The listing builds one solid part. Answer for the finished solid, in the listing's coordinates (mm). A direction names the side the tool comes from. Coordinates: 2 decimals unless noted, no trailing zeros. Write each loop counter-clockwise with the first axis right and the second up, starting at its lowest first coordinate (ties: lowest second). Pieces come first, ordered by that corner, then holes.
(1) The part is cut by section A-A on z = 11. Determine the outline of the cut face in (x, y), plus the area to 3 significant figures.
(2) Given P1, Ø5, axis at x = 0, z = 22.5, coming from the -Y side; P2, Ø3, axis at y = 1, z = 14, coming from the +X side; P3, Ø6, axis at x = 0.5, z = 16.5, coming from the -Y side, each flat-ended and moving along its own axis, determine where each tip first touches the part or whether it passes through.
(3) The part is cut by section C-C on y = -5. Determine the outline of the cut face in (x, z).
(4) The part is cut by section B-B on x = 0. Give the number of separate pieces and of enclosed holes in the cut face, plus the area to 3 significant figures.
(5) For a pull along Z with two mould halves and no side action, classify faces 6 (the flat face through (6.844, -3.774, 23.011)), 7 (the flat face through (3, -1.5, 3)), 8 (the flat face through (-6.4, 3.5, 9.6)), 9 (the flat face through (0, -1, 26)) as +Z half, -Z half, draft (parallel to the pull), parting line (faces both ways), or undercut.
(6) Straight lines are drawn through the part: line 1 (X direction, y = 2.75, z = 11); line 2 (X direction, y = 1.35, z = 19); line 3 (Z direction, x = 2.25, y = -0.5). For each, find the intervals that lie inside material, in ascending order.
(7) Which of the six approach directions +Z, -Z, +X, -X, +Y, -Y give full straight-line access (tool end or side, diameter ignored) to faces 1 (the flat face through (-3, 2, 24)), 2 (the flat face through (7.4, 1.5, 16.5)), 3 (the flat face through (7, -4, 23.8)), 4 (the conical face through (-7.37, 3.51, 18.09)), 5 (the flat face through (-3.76, -3.77, 24.92))?
from build123d import *
from build123d.topology import SkipClean

# Parameters (mm, degrees)
EXTRUDE_1_DEPTH        = 4
EXTRUDE_3_DEPTH        = 6
CHAMFER_1_SIZE         = 3
SKETCH_5_R             = 0.85
CUT_EXTRUDE_1_DEPTH    = 4
PATTERN_LINEAR_1_COUNT = 2
PATTERN_LINEAR_1_PITCH = 8
CUT_EXTRUDE_2_DEPTH    = 2.5
CUT_EXTRUDE_3_REACH    = 30.061
SKETCH_7_R             = 1.35
SKETCH_8_R             = 6
EXTRUDE_4_DEPTH        = 1.5
FILLET_1_R             = 0.5
SKETCH_9_R             = 5
CUT_EXTRUDE_4_DEPTH    = 3.6
SKETCH_10_R            = 3.55
CUT_EXTRUDE_5_DEPTH    = 3.6
CUT_EXTRUDE_6_DEPTH    = 0.8
CUT_EXTRUDE_7_DEPTH    = 29.786455148
FILLET_2_R             = 2
CHAMFER_2_SIZE         = 1


with BuildPart() as part:
    # ｽｹｯﾁ1 → ﾎﾞｽ - 押し出し1 (new body)
    with BuildSketch(Plane(origin=(0, 0, 0), x_dir=(1, 0, 0), z_dir=(0, 1, 0))):
        with BuildLine():
            Line((-7.9, 0), (-7.9, -26))
            Line((-7.9, -26), (7.9, -26))
            Line((7.9, -26), (7.9, 0))
            ThreePointArc((7.9, 0), (0, 7.9), (-7.9, 0))
        make_face()
    extrude(amount=EXTRUDE_1_DEPTH)

    # ｽｹｯﾁ4 → ﾎﾞｽ - 押し出し3 (add)
    with BuildSketch(Plane.XY.offset(26)):
        Polygon((-7, -5.5), (-4.5, -5.5), (-3, -2), (3, -2), (4.5, -5.5), (7, -5.5), (7.9, -2), (7.9, 0), (-7.9, 0), (-7.9, -2), align=None)
    extrude(amount=-EXTRUDE_3_DEPTH)

    # 面取り1
    chamfer_1_edges = [part.edges().sort_by_distance(p)[0] for p in [
        (0, 4, 26),
    ]]
    chamfer(chamfer_1_edges, length=CHAMFER_1_SIZE)

    # ｽｹｯﾁ5 → ｶｯﾄ - 押し出し1 (cut)
    with BuildSketch(Plane(origin=(0, 4, 0), x_dir=(1, 0, 0), z_dir=(0, 1, 0))):
        with Locations(Location((-4, -19, 0), (0, 0, 270))):
            Circle(SKETCH_5_R)
        with Locations(Location((4, -19, 0), (0, 0, 270))):
            Circle(SKETCH_5_R)
    cut_extrude_1 = extrude(amount=-CUT_EXTRUDE_1_DEPTH, mode=Mode.SUBTRACT)

    # 直線ﾊﾟﾀｰﾝ1: ｶｯﾄ - 押し出し1 ×2
    with Locations(*[(0, 0, -i * PATTERN_LINEAR_1_PITCH) for i in range(1, PATTERN_LINEAR_1_COUNT)]):
        add(cut_extrude_1, mode=Mode.SUBTRACT)

    # ｽｹｯﾁ6 → ｶｯﾄ - 押し出し2 (cut)
    with BuildSketch(Plane(origin=(0, 4, 0), x_dir=(1, 0, 0), z_dir=(0, 1, 0))):
        with BuildLine():
            Line((-3, -23), (-3, -27))
            Line((-3, -27), (3, -27))
            Line((3, -27), (3, -23))
            ThreePointArc((3, -23), (0, -20), (-3, -23))
        make_face()
    extrude(amount=-CUT_EXTRUDE_2_DEPTH, mode=Mode.SUBTRACT)

    # ｽｹｯﾁ7 → ｶｯﾄ - 押し出し3 (cut, up to next)
    with BuildSketch(Plane(origin=(0, 1.5, 0), x_dir=(1, 0, 0), z_dir=(0, 1, 0)), mode=Mode.PRIVATE) as cut_extrude_3_sk1:
        with Locations(Location((0, -23, 0), (0, 0, 270))):
            Circle(SKETCH_7_R)
    cut_extrude_3_tool1 = extrude(cut_extrude_3_sk1.sketch, amount=-CUT_EXTRUDE_3_REACH, mode=Mode.PRIVATE) & part.part
    add(cut_extrude_3_tool1.solids().sort_by_distance((0, 1.5, 23))[0], mode=Mode.SUBTRACT)

    # ｽｹｯﾁ8 → ﾎﾞｽ - 押し出し4 (add)
    with BuildSketch(Plane.XZ):
        with Locations(Location((0, 0, 0), (0, 0, 90))):
            Circle(SKETCH_8_R)
    extrude(amount=EXTRUDE_4_DEPTH)

    # ﾌｨﾚｯﾄ1
    fillet_1_edges = [part.edges().sort_by_distance(p)[0] for p in [
        (0, 0, -6),
    ]]
    fillet(fillet_1_edges, radius=FILLET_1_R)

    # ｽｹｯﾁ9 → ｶｯﾄ - 押し出し4 (cut)
    with BuildSketch(Plane(origin=(0, 4, 0), x_dir=(1, 0, 0), z_dir=(0, 1, 0))):
        with Locations(Location((0, 0, 0), (0, 0, 270))):
            Circle(SKETCH_9_R)
    extrude(amount=-CUT_EXTRUDE_4_DEPTH, mode=Mode.SUBTRACT)

    # ｽｹｯﾁ10 → ｶｯﾄ - 押し出し5 (cut)
    with BuildSketch(Plane(origin=(0, 0.4, 0), x_dir=(1, 0, 0), z_dir=(0, 1, 0))):
        with Locations(Location((0, 0, 0), (0, 0, 270))):
            Circle(SKETCH_10_R)
    extrude(amount=-CUT_EXTRUDE_5_DEPTH, mode=Mode.SUBTRACT)

    # ｽｹｯﾁ11 → ｶｯﾄ - 押し出し6 (cut, symmetric)
    with BuildSketch(Plane.XY.offset(23)):
        Polygon((3, -2), (4.5, -5.5), (5.1, -5.5), (3.6, -2), align=None)
        Polygon((7.9, -2), (7, -5.5), (6.4, -5.5), (7.3, -2), align=None)
    cut_extrude_6 = extrude(amount=CUT_EXTRUDE_6_DEPTH, both=True, mode=Mode.SUBTRACT)

    # ﾐﾗｰ1: ｶｯﾄ - 押し出し6 across plane
    add(cut_extrude_6.mirror(Plane(origin=(0, 0, 0), x_dir=(0, 0, 1), z_dir=(1, 0, 0))), mode=Mode.SUBTRACT)

    # ｽｹｯﾁ12 → ｶｯﾄ - 押し出し7 (cut, through all)
    with SkipClean():  # the faces are left unmerged after this step: merging them gives an invalid solid
        with BuildSketch(Plane(origin=(0, 4, 0), x_dir=(1, 0, 0), z_dir=(0, 1, 0))):
            with BuildLine():
                Line((-7.9, -18), (-6.9, -15))
                Line((-6.9, -15), (-6.9, -3.847076812))
                ThreePointArc((-6.9, -3.847076812), (-7.645913941, -1.987460691), (-7.9, 0))
                Line((-7.9, 0), (-7.9, -18))
            make_face()
        cut_extrude_7 = extrude(amount=-CUT_EXTRUDE_7_DEPTH, mode=Mode.SUBTRACT)

    # ﾐﾗｰ2: ｶｯﾄ - 押し出し7 across plane
    with SkipClean():  # the faces are left unmerged after this step: merging them gives an invalid solid
        add(cut_extrude_7.mirror(Plane(origin=(0, 0, 0), x_dir=(0, 0, 1), z_dir=(1, 0, 0))), mode=Mode.SUBTRACT)

    # ﾌｨﾚｯﾄ2
    fillet_2_edges = [part.edges().sort_by_distance(p)[0] for p in [
        (-7.9, 2, 18),
        (-6.9, 2, 3.847076812),
        (-6.9, 2, 15),
        (7.9, 2, 18),
        (6.9, 2, 15),
        (6.9, 2, 3.847076812),
    ]]
    fillet(fillet_2_edges, radius=FILLET_2_R)

    # 面取り2
    # the kernel refuses this chamfer: 1 mm, written as the material it adds along each edge
    with BuildSketch(Plane(origin=(7.9, 0, 20), x_dir=(0, 0.02749587661058639, -0.9996219169112968), z_dir=(-1, 0, 0))) as chamfer_2_piece_1_section:
        Polygon((CHAMFER_2_SIZE * 0.999621916911, CHAMFER_2_SIZE * 0.0274958766106), (-CHAMFER_2_SIZE * 0.0274958766106, CHAMFER_2_SIZE * 0.999621916911), (0, 0), align=None)
    chamfer_2_piece_1 = extrude(amount=15.8, mode=Mode.PRIVATE)
    chamfer_2_piece_1 = chamfer_2_piece_1 - Plane(origin=(-4, -0.34097177, 19), x_dir=(0, 0, 1), z_dir=(0, 1, 0)) * Cylinder(0.85, 36, mode=Mode.PRIVATE)
    chamfer_2_piece_1 = chamfer_2_piece_1 - Plane(origin=(4, -0.34097177, 19), x_dir=(0, 0, 1), z_dir=(0, 1, 0)) * Cylinder(0.85, 36, mode=Mode.PRIVATE)
    add(chamfer_2_piece_1)
    # the kernel refuses this chamfer: 1 mm, written as the material it takes off along each edge
    with BuildSketch(Plane(origin=(-7.9, 4, 18.32455532), x_dir=(-0.027495876610586487, -0.9996219169112968, 0), z_dir=(0, 0, 1)), Plane(origin=(7.9, 4, 25.571682988), x_dir=(0.027495876610586487, -0.9996219169112968, 0), z_dir=(0, 0, -1))) as chamfer_2_2_piece_1:
        Polygon((CHAMFER_2_SIZE * 0.999621916911, CHAMFER_2_SIZE * 0.0274958766106), (-CHAMFER_2_SIZE * 0.0274958766106, CHAMFER_2_SIZE * 0.999621916911), (0, 0), align=None)
    extrude(amount=7.247127668, mode=Mode.SUBTRACT)
    with BuildSketch(Plane(origin=(0, 4, 0), x_dir=(1, 0, 0), z_dir=(0, 0, 1))) as chamfer_2_2_piece_2:
        Polygon((7.9, -CHAMFER_2_SIZE), (7.9 - CHAMFER_2_SIZE, 0), (7.9, 0), align=None)
    revolve(axis=Axis((0, 4, 0), (0, 1, 0)), revolution_arc=180, mode=Mode.SUBTRACT)
    with BuildSketch(Plane(origin=(-5.9, 4, 18.32455532), x_dir=(-1, 0, 0), z_dir=(0, 0, 1))) as chamfer_2_2_piece_3:
        Polygon((2, CHAMFER_2_SIZE), (2 - CHAMFER_2_SIZE, 0), (2, 0), align=None)
    revolve(axis=Axis((-5.9, 4, 18.32455532), (0, -1, 0)), revolution_arc=18.434948823, mode=Mode.SUBTRACT)
    with BuildSketch(Plane(origin=(-7.797366596, 4, 17.692099788), x_dir=(-0.026084878905720917, -0.9996219169112968, -0.008694959635240323), z_dir=(0.31622776601683844, 0, -0.9486832980505137))) as chamfer_2_2_piece_4:
        Polygon((CHAMFER_2_SIZE * 0.999621916911, -CHAMFER_2_SIZE * 0.0274958766106), (-CHAMFER_2_SIZE * 0.0274958766106, -CHAMFER_2_SIZE * 0.999621916911), (0, 0), align=None)
    extrude(amount=2.513167019, mode=Mode.SUBTRACT)
    with BuildSketch(Plane(origin=(-8.9, 4, 14.67544468), x_dir=(0.9486832980505138, 0, 0.31622776601683794), z_dir=(-0.31622776601683794, 0, 0.9486832980505138))) as chamfer_2_2_piece_5:
        Polygon((2, -CHAMFER_2_SIZE), (2 + CHAMFER_2_SIZE, 0), (2, 0), align=None)
    revolve(axis=Axis((-8.9, 4, 14.67544468), (0, 1, 0)), revolution_arc=18.434948823, mode=Mode.SUBTRACT)
    with BuildSketch(Plane(origin=(-6.9, 4, 14.67544468), x_dir=(-0.027495876610586487, -0.9996219169112968, 0), z_dir=(0, 0, -1))) as chamfer_2_2_piece_6:
        Polygon((CHAMFER_2_SIZE * 0.999621916911, -CHAMFER_2_SIZE * 0.0274958766106), (-CHAMFER_2_SIZE * 0.0274958766106, -CHAMFER_2_SIZE * 0.999621916911), (0, 0), align=None)
    extrude(amount=10.339548002, mode=Mode.SUBTRACT)
    with BuildSketch(Plane(origin=(-8.9, 4, 4.335896678), x_dir=(1, 0, 0), z_dir=(0, 0, 1))) as chamfer_2_2_piece_7:
        Polygon((2, -CHAMFER_2_SIZE), (2 + CHAMFER_2_SIZE, 0), (2, 0), align=None)
    revolve(axis=Axis((-8.9, 4, 4.335896678), (0, 1, 0)), revolution_arc=25.974390018, mode=Mode.SUBTRACT)
    with BuildSketch(Plane(origin=(8.9, 4, 4.335896678), x_dir=(-0.8989898989898989, 0, -0.43796936138745074), z_dir=(0.43796936138745074, 0, -0.8989898989898989))) as chamfer_2_2_piece_8:
        Polygon((2, -CHAMFER_2_SIZE), (2 + CHAMFER_2_SIZE, 0), (2, 0), align=None)
    revolve(axis=Axis((8.9, 4, 4.335896678), (0, 1, 0)), revolution_arc=25.974390018, mode=Mode.SUBTRACT)
    with BuildSketch(Plane(origin=(6.9, 4, 14.67544468), x_dir=(0.027495876610586487, -0.9996219169112968, 0), z_dir=(0, 0, -1))) as chamfer_2_2_piece_9:
        Polygon((CHAMFER_2_SIZE * 0.999621916911, CHAMFER_2_SIZE * 0.0274958766106), (-CHAMFER_2_SIZE * 0.0274958766106, CHAMFER_2_SIZE * 0.999621916911), (0, 0), align=None)
    extrude(amount=10.339548002, mode=Mode.SUBTRACT)
    with BuildSketch(Plane(origin=(8.9, 4, 14.67544468), x_dir=(-1, 0, 0), z_dir=(0, 0, -1))) as chamfer_2_2_piece_10:
        Polygon((2, -CHAMFER_2_SIZE), (2 + CHAMFER_2_SIZE, 0), (2, 0), align=None)
    revolve(axis=Axis((8.9, 4, 14.67544468), (0, 1, 0)), revolution_arc=18.434948823, mode=Mode.SUBTRACT)
    with BuildSketch(Plane(origin=(7.797366596, 4, 17.692099788), x_dir=(0.026084878905720917, -0.9996219169112968, -0.008694959635240323), z_dir=(-0.31622776601683844, 0, -0.9486832980505137))) as chamfer_2_2_piece_11:
        Polygon((CHAMFER_2_SIZE * 0.999621916911, CHAMFER_2_SIZE * 0.0274958766106), (-CHAMFER_2_SIZE * 0.0274958766106, CHAMFER_2_SIZE * 0.999621916911), (0, 0), align=None)
    extrude(amount=2.513167019, mode=Mode.SUBTRACT)
    with BuildSketch(Plane(origin=(5.9, 4, 18.32455532), x_dir=(0.9486832980505135, 0, -0.3162277660168389), z_dir=(-0.3162277660168389, 0, -0.9486832980505135))) as chamfer_2_2_piece_12:
        Polygon((2, CHAMFER_2_SIZE), (2 - CHAMFER_2_SIZE, 0), (2, 0), align=None)
    revolve(axis=Axis((5.9, 4, 18.32455532), (0, -1, 0)), revolution_arc=18.434948823, mode=Mode.SUBTRACT)
    with BuildSketch(Plane(origin=(0, 4, 0), x_dir=(0.898989898989899, 0, 0.4379693613874505), z_dir=(-0.4379693613874505, 0, 0.898989898989899))) as chamfer_2_2_piece_13:
        Polygon((7.9, -CHAMFER_2_SIZE), (7.9 - CHAMFER_2_SIZE, 0), (7.9, 0), align=None)
    revolve(axis=Axis((0, 4, 0), (0, 1, 0)), revolution_arc=25.974390018, mode=Mode.SUBTRACT)
    with BuildSketch(Plane(origin=(0, 4, 0), x_dir=(-0.898989898989899, 0, 0.4379693613874506), z_dir=(0.4379693613874506, 0, 0.898989898989899))) as chamfer_2_2_piece_14:
        Polygon((7.9, CHAMFER_2_SIZE), (7.9 - CHAMFER_2_SIZE, 0), (7.9, 0), align=None)
    revolve(axis=Axis((0, 4, 0), (0, -1, 0)), revolution_arc=25.974390018, mode=Mode.SUBTRACT)


solid = part.part
Model answer:
1. outline: (-6.9, 0) - (-4.85, 0) - (-4.85, 4) - (-5.9, 4) - (-6.9, 3) - close; (-3.15, 0) - (3.15, 0) - (3.15, 4) - (-3.15, 4) - close; (4.85, 0) - (6.9, 0) - (6.9, 3) - (5.9, 4) - (4.85, 4) - close
1. area: 40.6 mm2
2. P1: stops at y = -2
2. P2: stops at x = 7.07
2. P3: stops at y = -0.5
3. outline: (-7.13, 20) - (-4.29, 20) - (-4.29, 22.2) - (-4.89, 22.2) - (-4.89, 23.8) - (-4.29, 23.8) - (-4.29, 26) - (-7.13, 26) - (-7.13, 23.8) - (-6.53, 23.8) - (-6.53, 22.2) - (-7.13, 22.2) - close; (4.29, 20) - (7.13, 20) - (7.13, 22.2) - (6.53, 22.2) - (6.53, 23.8) - (7.13, 23.8) - (7.13, 26) - (4.29, 26) - (4.29, 23.8) - (4.89, 23.8) - (4.89, 22.2) - (4.29, 22.2) - close
4. separate pieces: 3
4. enclosed holes: 0
4. area: 91.6 mm2
5. face 6: undercut
5. face 7: draft
5. face 8: undercut
5. face 9: +Z half
6. line 1: x = -6.9 to -4.85, -3.15 to 3.15, 4.85 to 6.9
6. line 2: x = -7.9 to -4.85, -3.15 to 3.15, 4.85 to 7.9
6. line 3: z = -5.56 to -2.75, 2.75 to 5.56, 19.5 to 26
7. face 1: +Z, +Y
7. face 2: +X, +Y, -Y
7. face 3: +X, -Y
7. face 4: -X, +Y
7. face 5: +Z, -Z, -Y
